Verification items for the finished model (mm, model axes). A direction names the side the tool comes from. Give positions to 0.01 mm unless a question says otherwise; leave off trailing zeros. Loops run counter-clockwise (first coordinate to the right, second up) from the corner with the lowest first, then second, coordinate; pieces in that order, holes last. Notation, with made-up numbers: M 53,48 L 89,48 A20 ccw 89,62 Z; hole C 33.25,12 d1. An arc over 180 degrees is marked long. Answer in a Markdown table with one row per item.
```python
from build123d import *

# Parameters (mm, degrees)
F0_R     = 9.525
F1_DEPTH = 25.4
F3_DEPTH = 25.401
F4_DEPTH = 12.7
F6_DEPTH = 10.16


with BuildPart() as f1:
    # F0 (on Front) → F1 (new body)
    with BuildSketch(Plane.XZ):
        Circle(F0_R)
    extrude(amount=F1_DEPTH)

    # F2 (on Front) → F3 (cut, through all)
    with BuildSketch(Plane.XZ):
        with BuildLine():
            ThreePointArc((4.7625, 0), (3.367596, 3.367596), (0, 4.7625))
            ThreePointArc((0, 4.7625), (-3.367596, 3.367596), (-4.7625, 0))
            ThreePointArc((-4.7625, 0), (-3.367596, -3.367596), (0, -4.7625))
            ThreePointArc((0, -4.7625), (3.367596, -3.367596), (4.7625, 0))
        make_face()
    extrude(amount=F3_DEPTH, mode=Mode.SUBTRACT)

    # F2 (on Front) → F4 (cut)
    with BuildSketch(Plane.XZ):
        with BuildLine():
            Line((4.7625, 0), (4.7625, 4.7625))
            Line((4.7625, 4.7625), (0, 4.7625))
            ThreePointArc((0, 4.7625), (3.367596, 3.367596), (4.7625, 0))
        make_face()
        with BuildLine():
            ThreePointArc((-4.7625, 0), (-3.367596, 3.367596), (0, 4.7625))
            Line((0, 4.7625), (-4.7625, 4.7625))
            Line((-4.7625, 4.7625), (-4.7625, 0))
        make_face()
        with BuildLine():
            Line((4.7625, -4.7625), (4.7625, 0))
            ThreePointArc((4.7625, 0), (3.367596, -3.367596), (0, -4.7625))
            Line((0, -4.7625), (4.7625, -4.7625))
        make_face()
        with BuildLine():
            ThreePointArc((0, -4.7625), (-3.367596, -3.367596), (-4.7625, 0))
            Line((-4.7625, 0), (-4.7625, -4.7625))
            Line((-4.7625, -4.7625), (0, -4.7625))
        make_face()
    extrude(amount=F4_DEPTH, mode=Mode.SUBTRACT)

    # F5 (on face) → F6 (cut)
    with BuildSketch(Plane.XZ.offset(25.4)):
        Polygon((2.986736, 7.210618), (-2.986736, 7.210618), (-7.210618, 2.986736), (-7.210618, -2.986736), (-2.986736, -7.210618), (2.986736, -7.210618), (7.210618, -2.986736), (7.210618, 2.986736), align=None)
    extrude(amount=-F6_DEPTH, mode=Mode.SUBTRACT)


solid = f1.part
```
Item 1: Sectioned sample at B-B (y = -15.75). Record the cut outline in (x, z) (3 decimals).
Reported:
| item | result |
|---|---|
| outline | C 0,0 d19.05; hole M -7.211,-2.987 L -2.987,-7.211 L 2.987,-7.211 L 7.211,-2.987 L 7.211,2.987 L 2.987,7.211 L -2.987,7.211 L -7.211,2.987 Z |
Item 2: Release check for a two-part mould opening along X. For faces 4 (the flat face through (0, 0, -6)), 5 (the cylindrical face through (-7.559, -12.522, -5.796)), 6 (the flat face through (4.762, -6, 0)) record: released by +X, released by -X, zero draft, split by the parting line, or undercut.
Reported:
| item | result |
|---|---|
| face 4 | zero draft |
| face 5 | split by the parting line |
| face 6 | undercut |
Item 3: Scan lines: L1, parallel to Z at x = 0.25, y = -12.25; L2, parallel to X at y = -19.25, z = 4.5; L3, parallel to Z at x = 4.5, y = -6.75. Record each from-to range of solid material in increasing order. Write a range as [from, to].
Reported:
| item | result |
|---|---|
| L1 | z = [-9.52, -4.76], [4.76, 9.52] |
| L2 | x = [-8.39, -5.7], [5.7, 8.39] |
| L3 | z = [-8.39, -4.76], [4.76, 8.39] |
Item 4: Sectioned sample at A-A (z = 1.75). Record the cut outline in (x, y), and give its area (3 significant figures).
Reported:
| item | result |
|---|---|
| outline | M -9.36,-25.4 L -7.21,-25.4 L -7.21,-15.24 L -4.43,-15.24 L -4.43,-12.7 L -4.76,-12.7 L -4.76,0 L -9.36,0 Z; M 4.43,-15.24 L 7.21,-15.24 L 7.21,-25.4 L 9.36,-25.4 L 9.36,0 L 4.76,0 L 4.76,-12.7 L 4.43,-12.7 Z |
| area | 186 mm^2 |
Item 5: Go/stop test with flat-tipped pins: pin 1 (6 mm diameter, centred on x = -4, y = -15, fed in from +Z); pin 2 (6 mm diameter, centred on x = 6.5, y = -13, fed in from +Z); pin 3 (1 mm diameter, centred on y = -14.5, z = 4, fed in from -X). Record where each tip stops, or that it passes through.
Reported:
| item | result |
|---|---|
| pin 1 | stops at z = 9.47 |
| pin 2 | stops at z = 8.86 |
| pin 3 | stops at x = -8.86 |
Item 6: Tool access check on faces 1 (the flat face through (5, -25.4, 6)), 2 (the flat face through (0, -20, 7.211)), 3 (the flat face through (-4, -12.7, 4)). Record the directions out of +Z, -Z, +X, -X, +Y, -Y that give a thin tool (end or side, any length) a straight path to the whole face; none if there is none.
Reported:
| item | result |
|---|---|
| face 1 | +Z, -Z, +X, -X, -Y |
| face 2 | -Y |
| face 3 | +Y |
Item 7: Sectioned sample at C-C (x = 5.5). Record the cut outline in (y, z).
Reported:
| item | result |
|---|---|
| outline | M -25.4,-7.78 L 0,-7.78 L 0,7.78 L -25.4,7.78 L -25.4,4.7 L -15.24,4.7 L -15.24,-4.7 L -25.4,-4.7 Z |
Item 8: Sectioned sample at D-D (z = 6). Record the cut outline in (x, y), and give its area (3 significant figures).
Reported:
| item | result |
|---|---|
| outline | M -7.4,-25.4 L -4.2,-25.4 L -4.2,-15.24 L 4.2,-15.24 L 4.2,-25.4 L 7.4,-25.4 L 7.4,0 L -7.4,0 Z |
| area | 291 mm^2 |
